from build123d import *

# Parameters (mm, degrees)
SKETCH3_W           = 90
SKETCH3_H           = 50
BOSS_EXTRUDE4_DEPTH = 15
SKETCH4_W           = 60
SKETCH4_H           = 10
BOSS_EXTRUDE5_DEPTH = 25
SKETCH5_R           = 5
CUT_EXTRUDE1_DEPTH  = 79.262379212
FILLET1_SIZE        = 10


with BuildPart() as part:
    # Sketch3 → Boss-Extrude4 (new body)
    with BuildSketch(Plane.XY):
        Rectangle(SKETCH3_W, SKETCH3_H)
    extrude(amount=BOSS_EXTRUDE4_DEPTH)

    # Sketch4 → Boss-Extrude5 (add)
    with BuildSketch(Plane.XY.offset(15)):
        with Locations((0, 20)):
            Rectangle(SKETCH4_W, SKETCH4_H)
        with Locations((0, -20)):
            Rectangle(SKETCH4_W, SKETCH4_H)
    extrude(amount=BOSS_EXTRUDE5_DEPTH)

    # Sketch5 → Cut-Extrude1 (cut, through all)
    with BuildSketch(Plane.XZ.offset(25)):
        with Locations(Location((0, 27.5, 0), (0, 0, 270))):
            Circle(SKETCH5_R)
    extrude(amount=-CUT_EXTRUDE1_DEPTH, mode=Mode.SUBTRACT)

    # Fillet1
    fillet1_edges = [part.edges().sort_by_distance(p)[0] for p in [
        (-30, 20, 40),
        (30, 20, 40),
        (30, -20, 40),
        (-30, -20, 40),
    ]]
    chamfer(fillet1_edges, length=FILLET1_SIZE)


solid = part.part
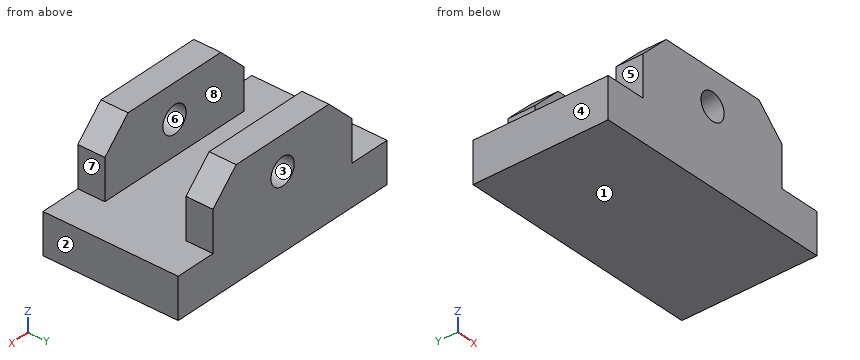
Input: part model. Units: mm. Frame: model coordinates. Face numbers are marked on the shaded views. A direction names the side the tool comes from. Give positions to 0.01 mm unless a question says otherwise; leave off trailing zeros. Write each loop counter-clockwise with the first axis right and the second up, starting at its lowest first coordinate (ties: lowest second). Pieces come first, ordered by that corner, then holes. Notation, with made-up numbers: (66, 84.5) -> (121, 84.5) arc R18 ccw to (121, 110.5) -> close; hole circle Ø6 at (88.5, 20). An arc over 180 degrees is marked (long way). Use one line per item in the form item = value. Start each with the question number.
1) Pin query (flat end, axial travel): pin 1 (8 mm diameter, centred on y = 14, z = 16, fed in from +X); pin 2 (8 mm diameter, centred on x = 0, z = 27.5, fed in from +Y); pin 3 (2 mm diameter, centred on x = 14, y = 3.5, fed in from +Z); pin 4 (5 mm diameter, centred on y = -20.5, z = 25.5, fed in from +X). Return the tip coordinate at first contact, or that it passes through.
2) Section query A-A on z = 27.5. Return the cut outline in (x, y), then the cut area to 3 significant figures.
3) Draft query along X for the marked faces 1, 2, 3 and 4. Return one class per face: pulls with the +X half, pulls with the -X half, needs draft (parallel to the pull), parting line crosses it, or undercut.
4) Set-up query: the marked faces 5, 6, 7 and 8. Return all of +Z, -Z, +X, -X, +Y, -Y with unobstructed straight access to the full face (end or side cutting, diameter ignored); none if empty.
5) Section query D-D on x = -27. Return the cut outline in (y, z), then the cut area to 3 significant figures.
6) Section query B-B on x = 0. Return the cut outline in (y, z).
7) Ray query, probe 1 along X at (y, z) = (17.75, 27.5); probe 2 along Y at (x, z) = (-16, 38); probe 3 along Z at (x, y) = (-30.5, -10.5). Return the intervals inside material, ascending. Write a range as from..to.
8) Section query C-C on y = -19.5. Return the cut outline in (x, z).
Outcome:
q1.pin_1 = 45
q1.pin_2 = through
q1.pin_3 = 15
q1.pin_4 = 30
q2.outline = (-30, -25) -> (-5, -25) -> (-5, -15) -> (-30, -15) -> close; (-30, 15) -> (-5, 15) -> (-5, 25) -> (-30, 25) -> close; (5, -25) -> (30, -25) -> (30, -15) -> (5, -15) -> close; (5, 15) -> (30, 15) -> (30, 25) -> (5, 25) -> close
q2.area = 1,000 mm^2
q3.face_1 = needs draft
q3.face_2 = pulls with the +X half
q3.face_3 = undercut
q3.face_4 = pulls with the -X half
q4.face_5 = +Z, -X, +Y, -Y
q4.face_6 = +Y, -Y
q4.face_7 = +Z, +X, +Y, -Y
q4.face_8 = +Z, +X, -X
q5.outline = (-25, 0) -> (25, 0) -> (25, 33) -> (15, 33) -> (15, 15) -> (-15, 15) -> (-15, 33) -> (-25, 33) -> close
q5.area = 1,110 mm^2
q6.outline = (-25, 0) -> (25, 0) -> (25, 22.5) -> (15, 22.5) -> (15, 15) -> (-15, 15) -> (-15, 22.5) -> (-25, 22.5) -> close; (-25, 32.5) -> (-15, 32.5) -> (-15, 40) -> (-25, 40) -> close; (15, 32.5) -> (25, 32.5) -> (25, 40) -> (15, 40) -> close
q7.probe_1 = -30..-5, 5..30
q7.probe_2 = -25..-15, 15..25
q7.probe_3 = 0..15
q8.outline = (-45, 0) -> (45, 0) -> (45, 15) -> (30, 15) -> (30, 30) -> (20, 40) -> (-20, 40) -> (-30, 30) -> (-30, 15) -> (-45, 15) -> close; hole circle Ø10 at (0, 27.5)
